Work out the finished part from the listing and answer in its coordinate system (mm). Face numbers are marked on the shaded views. A direction names the side the tool comes from. Coordinates: 2 decimals unless noted, no trailing zeros. Loops run counter-clockwise (first coordinate to the right, second up) from the corner with the lowest first, then second, coordinate; pieces in that order, holes last. Notation, with made-up numbers: M 79.25,87.5 L 98.25,87.5 A19 cw 98.25,113.5 Z; hole C 32,-10 d5. An arc over 180 degrees is marked long. Write each question's results on one line, items separated by ' | '.
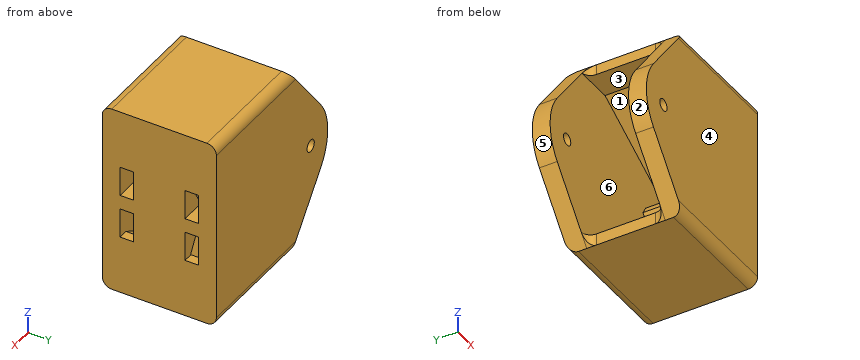
```python
from build123d import *

# Parameters (mm, degrees)
BOSS_EXTRUDE2_DEPTH = 3.3
SKETCH5_R           = 0.5
SKETCH5_W           = 10.292404403
SKETCH5_H           = 16
BOSS_EXTRUDE3_DEPTH = 1.5
SKETCH7_W           = 2.4988973
SKETCH7_H           = 1.136262802
CUT_EXTRUDE1_DEPTH  = 18.9628088
FILLET1_R           = 0.8
FILLET2_R           = 0.8


with BuildPart() as part:
    # Sketch6 → Boss-Extrude2 (new, symmetric)
    with BuildSketch(Plane(origin=(0, 0, 0), x_dir=(1, 0, 0), z_dir=(0, 1, 0))):
        Polygon((13, 8), (13, -8), (4.706393415, -8), (2.707595597, -8), (2.707595597, -7.141772619), (5.22657427, -7.141772619), (12.244932652, -3.06812199), (10.464109218, 0), (12.244932652, 3.06812199), (5.438439019, 7.01880042), (2.707595597, 7.01880042), (2.707595597, 8), (4.706393415, 8), align=None)
    extrude(amount=BOSS_EXTRUDE2_DEPTH, both=True)

    # Sketch5 → Boss-Extrude3 (add)
    # profile 1 of 2: a face of its own
    with BuildSketch(Plane(origin=(0, 3.3, 0), x_dir=(1, 0, 0), z_dir=(0, 1, 0))):
        with BuildLine():
            Line((2.707595597, -8), (2.707595597, 8))
            Line((2.707595597, 8), (-1.374953719, 2.814641346))
            ThreePointArc((-1.374953719, 2.814641346), (-2.35, 0), (-1.374953719, -2.814641346))
            Line((-1.374953719, -2.814641346), (2.707595597, -8))
        make_face()
        with Locations(Location((0, 0, 0), (0, 0, 270))):
            Circle(SKETCH5_R, mode=Mode.SUBTRACT)
    # profile 2 of 2: a face of its own
    with BuildSketch(Plane(origin=(0, 3.3, 0), x_dir=(1, 0, 0), z_dir=(0, 1, 0))):
        with Locations((7.853797799, 0)):
            Rectangle(SKETCH5_W, SKETCH5_H)
    boss_extrude3 = extrude(amount=BOSS_EXTRUDE3_DEPTH)

    # Mirror1: Boss-Extrude3 across plane
    add(boss_extrude3.mirror(Plane.ZX))

    # Sketch7 → Cut-Extrude1 (cut, through all)
    with BuildSketch(Plane(origin=(13, 0, 0), x_dir=(0, 0, -1), z_dir=(1, 0, 0))):
        with Locations((-1.85055135, 2.731868599)):
            Rectangle(SKETCH7_W, SKETCH7_H)
        with Locations((1.85055135, 2.731868599)):
            Rectangle(SKETCH7_W, SKETCH7_H)
        with Locations((-1.85055135, -2.731868599)):
            Rectangle(SKETCH7_W, SKETCH7_H)
        with Locations((1.85055135, -2.731868599)):
            Rectangle(SKETCH7_W, SKETCH7_H)
    extrude(amount=-CUT_EXTRUDE1_DEPTH, mode=Mode.SUBTRACT)

    # Fillet1
    # the kernel refuses this fillet: 0.8 mm, written as the material it adds along each edge
    with BuildSketch(Plane(origin=(2.707595597, -3.3, 8), x_dir=(0, 1, 0), z_dir=(0, 0, -1))) as fillet1_piece_1_section:
        with BuildLine():
            CenterArc((FILLET1_R, -FILLET1_R), FILLET1_R, 90, 90)
            Line((0, -FILLET1_R), (0, 0))
            Line((0, 0), (FILLET1_R, 0))
        make_face()
    fillet1_piece_1 = extrude(amount=0.858227381, mode=Mode.PRIVATE)
    fillet1_piece_1 = split(fillet1_piece_1, bisect_by=Plane(origin=(2.414269103, -3.083958399, 7.627437917), z_dir=(0.785704114090993, 0, -0.6186024936099819)), keep=Keep.TOP, mode=Mode.PRIVATE)
    add(fillet1_piece_1)
    with BuildSketch(Plane(origin=(2.707595597, -3.3, -7.01880042), x_dir=(0, 1, 0), z_dir=(0, 0, -1))) as fillet1_piece_2_section:
        with BuildLine():
            CenterArc((FILLET1_R, -FILLET1_R), FILLET1_R, 90, 90)
            Line((0, -FILLET1_R), (0, 0))
            Line((0, 0), (FILLET1_R, 0))
        make_face()
    fillet1_piece_2 = extrude(amount=0.98119958, mode=Mode.PRIVATE)
    fillet1_piece_2 = split(fillet1_piece_2, bisect_by=Plane(origin=(2.378311496, -3.089381115, -7.581767168), z_dir=(0.7857041140909933, 0, 0.6186024936099818)), keep=Keep.TOP, mode=Mode.PRIVATE)
    add(fillet1_piece_2)
    with BuildSketch(Plane(origin=(2.707595597, 3.3, -7.01880042), x_dir=(0, -1, 0), z_dir=(0, 0, -1))) as fillet1_piece_3_section:
        with BuildLine():
            CenterArc((FILLET1_R, FILLET1_R), FILLET1_R, 180, 90)
            Line((0, FILLET1_R), (0, 0))
            Line((0, 0), (FILLET1_R, 0))
        make_face()
    fillet1_piece_3 = extrude(amount=0.98119958, mode=Mode.PRIVATE)
    fillet1_piece_3 = split(fillet1_piece_3, bisect_by=Plane(origin=(2.378311496, 3.089381115, -7.581767168), z_dir=(0.7857041140909933, 0, 0.6186024936099818)), keep=Keep.TOP, mode=Mode.PRIVATE)
    add(fillet1_piece_3)
    with BuildSketch(Plane(origin=(2.707595597, 3.3, 8), x_dir=(0, -1, 0), z_dir=(0, 0, -1))) as fillet1_piece_4_section:
        with BuildLine():
            CenterArc((FILLET1_R, FILLET1_R), FILLET1_R, 180, 90)
            Line((0, FILLET1_R), (0, 0))
            Line((0, 0), (FILLET1_R, 0))
        make_face()
    fillet1_piece_4 = extrude(amount=0.858227381, mode=Mode.PRIVATE)
    fillet1_piece_4 = split(fillet1_piece_4, bisect_by=Plane(origin=(2.414269103, 3.083958399, 7.627437917), z_dir=(0.785704114090993, 0, -0.6186024936099819)), keep=Keep.TOP, mode=Mode.PRIVATE)
    add(fillet1_piece_4)

    # Fillet2
    fillet2_edges = [part.edges().sort_by_distance(p)[0] for p in [
        (7.853797799, 4.8, 8),
        (7.853797799, 4.8, -8),
        (7.853797799, -4.8, -8),
        (7.853797799, -4.8, 8),
    ]]
    fillet(fillet2_edges, radius=FILLET2_R)


solid = part.part
```
1) Find section B-B, the plane z = -1.5. Give the vertices of the cut face in (x, y), and give its area (3 significant figures).
Check result:
outline: M -2.1,-4.8 L 13,-4.8 L 13,-3.3 L -2.1,-3.3 Z; M -2.1,3.3 L 13,3.3 L 13,4.8 L -2.1,4.8 Z; M 11.33,-2.16 L 13,-2.16 L 13,2.16 L 11.33,2.16 Z | area: 52.5 mm^2
2) Find section A-A, the plane x = 0. Give the vertices of the cut face in (y, z).
Check result:
outline: M -4.8,-4.56 L -3.3,-4.56 L -3.3,-0.5 L -4.8,-0.5 Z; M -4.8,0.5 L -3.3,0.5 L -3.3,4.56 L -4.8,4.56 Z; M 3.3,-4.56 L 4.8,-4.56 L 4.8,-0.5 L 3.3,-0.5 Z; M 3.3,0.5 L 4.8,0.5 L 4.8,4.56 L 3.3,4.56 Z
3) For a pull along Z with two mould halves and no side action, classify the marked faces 1, 2, 3 and 4 as released by +Z, released by -Z, zero draft, split by the parting line, or undercut.
Check result:
face 1: undercut | face 2: split by the parting line | face 3: undercut | face 4: zero draft
4) Given pin 1 Ø0.8 at (y, z) = (0.5, -7.5) entering from -X; pin 2 Ø2 at (y, z) = (1.5, -5.5) entering from -X, each flat-ended and moving along its own axis, determine where each tip first touches the part or whether it passes through.
Check result:
pin 1: x = 2.71 | pin 2: x = 6.33
5) Find section D-D, the plane y = 0. Give the vertices of the cut face in (x, z).
Check result:
outline: M 2.71,-8 L 13,-8 L 13,8 L 2.71,8 L 2.71,7.14 L 5.23,7.14 L 12.24,3.07 L 10.46,0 L 12.24,-3.07 L 5.44,-7.02 L 2.71,-7.02 Z
6) Straight lines are drawn through the part: probe 1 along Y at (x, z) = (11.25, -0.75); probe 2 along Y at (x, z) = (9.25, 4); probe 3 along X at (y, z) = (4.35, 0). For each, find the intervals that lie inside material, in ascending order. Write a range as [from, to].
Check result:
probe 1: [-4.8, -3.3], [-2.16, 2.16], [3.3, 4.8] | probe 2: [-4.8, -3.3], [3.3, 4.8] | probe 3: [-2.35, -0.5], [0.5, 13]
7) Which of the six approach directions +Z, -Z, +X, -X, +Y, -Y give full straight-line access (tool end or side, diameter ignored) to the marked faces 5 and 6?
Check result:
face 5: -X, +Y, -Y | face 6: -X
8) Find section C-C, the plane y = -3.75. Give the vertices of the cut face in (x, z).
Check result:
outline: M -1.37,-2.81 L 2.71,-8 L 13,-8 L 13,8 L 2.71,8 L -1.37,2.81 A4.55 ccw Z; hole C 0,0 d1
